Design review of the part built by this model. Coordinates are the model's own, in mm. A direction names the side the tool comes from. Round coordinates to 2 decimals unless told otherwise and drop trailing zeros. Write each loop counter-clockwise with the first axis right and the second up, starting at its lowest first coordinate (ties: lowest second). Pieces come first, ordered by that corner, then holes. Notation, with made-up numbers: M 48.5,-22.5 L 80.5,-22.5 A16 ccw 80.5,-7.5 Z; hole C 73,78.25 d10. An arc over 180 degrees is marked long. One line per question, with ' | ' between items. Start each with the question number.
Item 1: Add section B-B, the plane z = 18.5. State the section outline as (x, y) points, and give its area (3 significant figures).
Item 2: Add section D-D, the plane x = -57. State the section outline as (y, z) points, and give its area (3 significant figures).
Item 3: Draft analysis for pull direction X (two halves, no side actions). For faces 1 (the face through (55.282, 13, 31)), 2 (the face through (-11, 13, 0)), 3 (the face through (-9, 13, -4)), state which applies: released by +X, released by -X, zero draft, split by the parting line, or undercut.
Item 4: Add section A-A, the plane y = 12.7. State the section outline as (x, z) points.
Item 5: For L1, parallel to X at y = 11.5, z = 31.5; L2, parallel to Z at x = 12, y = 11.25, list the stretches that pass through material, from the lowest coordinate up.
Item 6: Add section C-C, the plane z = 56. State the section outline as (x, y) points.
Item 7: Machinability: for faces 4 (the face through (-71.718, 13, 33)), 5 (the face through (-15.4, 0, -0.3)), which of the approach directions +Z, -Z, +X, -X, +Y, -Y give a long, thin tool a straight path to every point of the face, cutting with its end or side? Answer none if there is none.
Item 8: Insertion check: pin 1 Ø6 at (y, z) = (12.7, 56.97) entering from +X; pin 2 Ø6 at (x, y) = (-7, 3) entering from +Z; pin 3 Ø4 at (y, z) = (12.7, 56.97) entering from -X. Each pin has a flat end and moves straight along its axis. Give the tip position at first contact, or say it passes through.
```python
from build123d import *

# Parameters (mm, degrees)
SALIENTE_EXTRUIR1_DEPTH    = 25.4
CROQUIS3_R                 = 2.5
CORTAR_EXTRUIR1_DEPTH      = 1
CORTAR_EXTRUIR1_DEPTH_BACK = 132


with BuildPart() as part:
    # Croquis1 → Saliente-Extruir1 (new body)
    with BuildSketch(Plane(origin=(0, 0, 0), x_dir=(1, 0, 0), z_dir=(0, 1, 0))):
        Polygon((-71.71783911, 0), (51.28216089, 0), (51.28216089, -65), (55.28216089, -65), (55.28216089, 4), (-75.71783911, 4), (-75.71783911, -65), (-71.71783911, -65), align=None)
    extrude(amount=SALIENTE_EXTRUIR1_DEPTH)

    # Croquis3 → Cortar-Extruir1 (cut, two sides)
    with BuildSketch(Plane(origin=(55.28216089, 0, 0), x_dir=(0, 0, -1), z_dir=(1, 0, 0))) as cortar_extruir1_sk:
        with Locations((-56.969231592, 12.7)):
            Circle(CROQUIS3_R)
    extrude(amount=CORTAR_EXTRUIR1_DEPTH, mode=Mode.SUBTRACT)
    extrude(cortar_extruir1_sk.sketch, amount=-CORTAR_EXTRUIR1_DEPTH_BACK, mode=Mode.SUBTRACT)


solid = part.part
```
Computed values:
1) outline: M -75.72,0 L -71.72,0 L -71.72,25.4 L -75.72,25.4 Z; M 51.28,0 L 55.28,0 L 55.28,25.4 L 51.28,25.4 Z | area: 203 mm^2
2) outline: M 0,-4 L 25.4,-4 L 25.4,0 L 0,0 Z | area: 102 mm^2
3) face 1: released by +X | face 2: undercut | face 3: zero draft
4) outline: M -75.72,-4 L 55.28,-4 L 55.28,54.47 L 51.28,54.47 L 51.28,0 L -71.72,0 L -71.72,54.47 L -75.72,54.47 Z; M -75.72,59.47 L -71.72,59.47 L -71.72,65 L -75.72,65 Z; M 51.28,59.47 L 55.28,59.47 L 55.28,65 L 51.28,65 Z
5) L1: x = -75.72 to -71.72, 51.28 to 55.28 | L2: z = -4 to 0
6) outline: M -75.72,0 L -71.72,0 L -71.72,10.4 L -75.72,10.4 Z; M -75.72,15 L -71.72,15 L -71.72,25.4 L -75.72,25.4 Z; M 51.28,0 L 55.28,0 L 55.28,10.4 L 51.28,10.4 Z; M 51.28,15 L 55.28,15 L 55.28,25.4 L 51.28,25.4 Z
7) face 4: +Z, +Y, -Y | face 5: +Z, -Z, +X, -X, -Y
8) pin 1: stops at x = 55.28 | pin 2: stops at z = 0 | pin 3: passes through
